Drawing for the job (mm, zero at the part's lowest x, y, z). A direction names the side the tool comes from. Coordinates: 2 decimals unless noted, no trailing zeros. Write each loop counter-clockwise with the first axis right and the second up, starting at its lowest first coordinate (ties: lowest second). Pieces come first, ordered by that corner, then holes. Notation, with made-up numbers: M 38.5,-5 L 76.5,-5 A21 cw 76.5,4 Z; hole C 88,54 d3. An arc over 180 degrees is marked long. Put each result on its own line as item: value. Start each with the question number.
Q1. Cut at D-D (z = 22). Write the cut outline in (x, y), then the cut area to 3 significant figures.
Q2. Drill centre lines: line 1 along Y through (x, z) = (4.7, 9.5); line 2 along Z through (x, y) = (2.75, 7.5); line 3 along Y through (x, z) = (5.75, 11). Where is each one in solid material? Low to high.
Q3. Which spindle directions (+Z, -Z, +X, -X, +Y, -Y) get a long thin tool onto all of the face, cutting with end or side? Do the marked faces 1 and 2. Say none if no direction does.
Q4. Cut at A-A (y = 4.7). Write the cut outline in (x, z).
Q5. Drop flat-ended pins along their axis: pin 1 (2 mm diameter, centred on y = 8, z = 21.5, fed in from +X); pin 2 (5 mm diameter, centred on y = 2, z = 20.5, fed in from +X) (3 decimals). Give the stop position or say it passes through.
Q6. Cut at C-C (y = 2.25). Write the cut outline in (x, z), then the cut area to 3 significant figures.
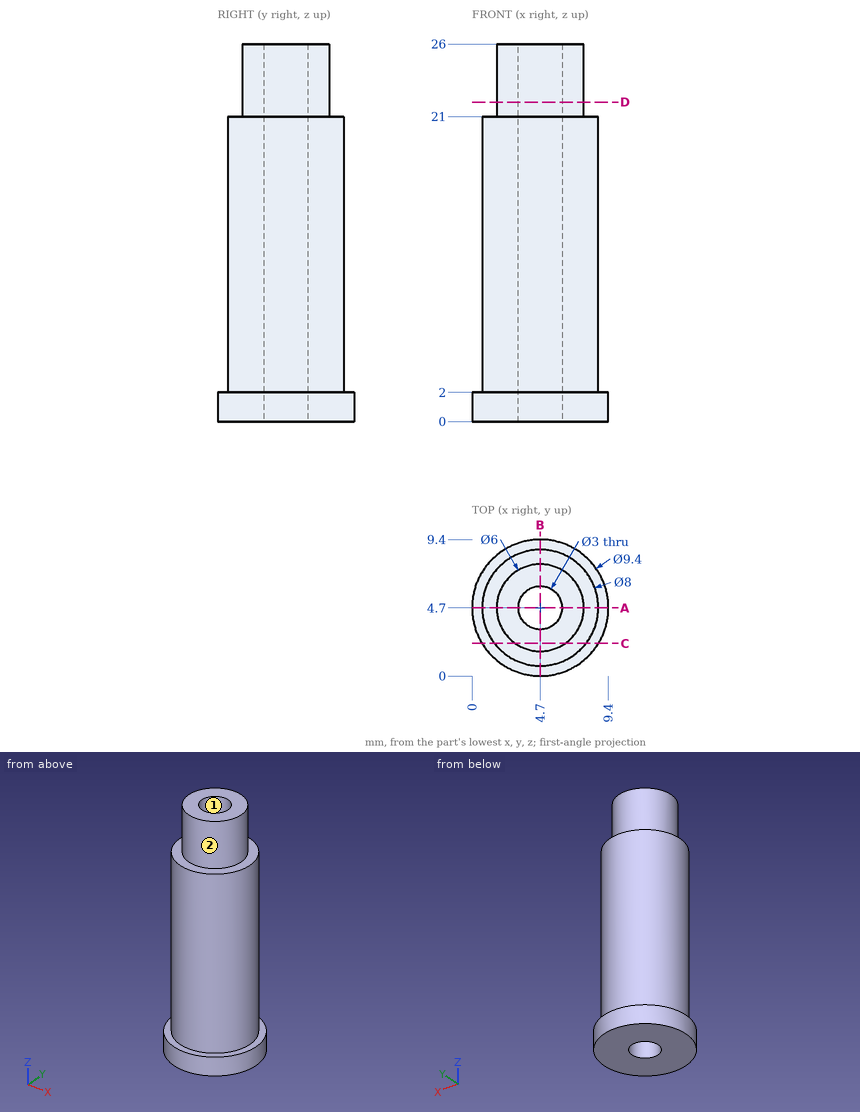
Computed values:
1. outline: C 4.7,4.7 d6; hole C 4.7,4.7 d3
1. area: 21.2 mm2
2. line 1: 0.7 to 3.2, 6.2 to 8.7
2. line 2: 0 to 21
2. line 3: 0.84 to 3.63, 5.77 to 8.56
3. face 1: +Z, -Z
3. face 2: +Z
4. outline: M 0,0 L 3.2,0 L 3.2,26 L 1.7,26 L 1.7,21 L 0.7,21 L 0.7,2 L 0,2 Z; M 6.2,0 L 9.4,0 L 9.4,2 L 8.7,2 L 8.7,21 L 7.7,21 L 7.7,26 L 6.2,26 Z
5. pin 1: x = 7.87
5. pin 2: x = 8.695
6. outline: M 0.69,0 L 8.71,0 L 8.71,2 L 7.86,2 L 7.86,21 L 6.43,21 L 6.43,26 L 2.97,26 L 2.97,21 L 1.54,21 L 1.54,2 L 0.69,2 Z
6. area: 154 mm2
